Answer from the drawing. Dimensions are ordinates in mm from the lowest x, y and z of the part. Round coordinates to 2 decimals unless told otherwise and drop trailing zeros. Order: outer loops, then holes, each group sorted by start corner. A loop starts at its lowest first (then second) coordinate and runs counter-clockwise, first axis right, second up. Notation, with made-up numbers: (28, 61.25) -> (36, 61.25) arc R16 cw to (36, 69.25) -> close; hole circle Ø10 at (-3, 17.25). An arc over 180 degrees is marked (long way). Use a Markdown table: item, result. Add a question column.
1. Section A-A, the plane z = 200 is taken. Give the vertices of the cut face in (x, y).
2. Section D-D, the plane x = 110 is taken. Give the vertices of the cut face in (y, z).
3. Consider L1, parallel to Z at x = 170, y = 31; L2, parallel to X at y = 19, z = 229; L3, parallel to X at y = 29, z = 200. Determine where each line is inside the solid, lowest interval first. Write a range as [from, to].
4. Section B-B, the plane y = 16.5 is taken. Give the vertices of the cut face in (x, z).
5. Section C-C, the plane x = 50 is taken. Give the vertices of the cut face in (y, z), then the cut area to 3 significant figures.
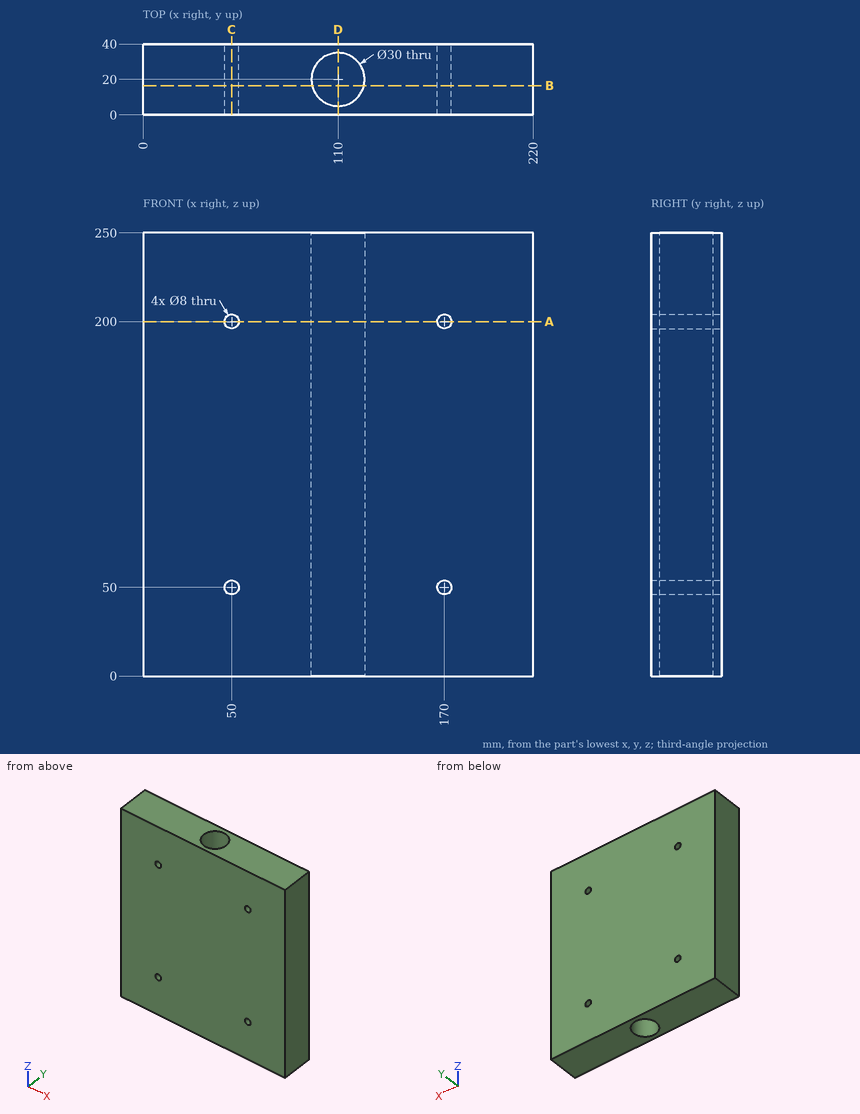
Verdict:
| question | item | result |
|---|---|---|
| 1 | outline | (0, 0) -> (46, 0) -> (46, 40) -> (0, 40) -> close; (54, 0) -> (166, 0) -> (166, 40) -> (54, 40) -> close; (174, 0) -> (220, 0) -> (220, 40) -> (174, 40) -> close; hole circle Ø30 at (110, 20) |
| 2 | outline | (0, 0) -> (5, 0) -> (5, 250) -> (0, 250) -> close; (35, 0) -> (40, 0) -> (40, 250) -> (35, 250) -> close |
| 3 | L1 | z = [0, 46], [54, 196], [204, 250] |
| 3 | L2 | x = [0, 95.03], [124.97, 220] |
| 3 | L3 | x = [0, 46], [54, 98], [122, 166], [174, 220] |
| 4 | outline | (0, 0) -> (95.41, 0) -> (95.41, 250) -> (0, 250) -> close; (124.59, 0) -> (220, 0) -> (220, 250) -> (124.59, 250) -> close; hole circle Ø8 at (50, 50); hole circle Ø8 at (50, 200); hole circle Ø8 at (170, 50); hole circle Ø8 at (170, 200) |
| 5 | outline | (0, 0) -> (40, 0) -> (40, 46) -> (0, 46) -> close; (0, 54) -> (40, 54) -> (40, 196) -> (0, 196) -> close; (0, 204) -> (40, 204) -> (40, 250) -> (0, 250) -> close |
| 5 | area | 9,360 mm2 |
